```python
from build123d import *

# Parameters (mm, degrees)
SKETCH1_R           = 8
BOSS_EXTRUDE1_DEPTH = 55.781202295
BOSS_EXTRUDE2_DEPTH = 7.5
SKETCH4_W           = 9
SKETCH4_H           = 15
FILLET7_R           = 7.5


with BuildPart() as part:
    # Sketch1 → Boss-Extrude1 (new body)
    with BuildSketch(Plane.XY):
        with Locations(Location((0, 0, 0), (0, 0, 180))):
            Circle(SKETCH1_R)
    extrude(amount=BOSS_EXTRUDE1_DEPTH)

    # Sketch2 → Boss-Extrude2 (add, symmetric)
    with BuildSketch(Plane(origin=(0, 0, 0), x_dir=(1, 0, 0), z_dir=(0, 1, 0))):
        with BuildLine():
            Line((0, 0), (0, -47.781202295))
            Line((0, -47.781202295), (-8, -47.781202295))
            ThreePointArc((-8, -47.781202295), (-15.893349065, -27.087541453), (-35.563103488, -16.907496293))
            ThreePointArc((-35.563103488, -16.907496293), (-57.085036764, -8.603159393), (-71.811764706, 9.152941176))
            Line((-71.811764706, 9.152941176), (-78.588235294, 23.647058824))
            ThreePointArc((-78.588235294, 23.647058824), (-71.352941176, 43.588235294), (-51.411764706, 36.352941176))
            ThreePointArc((-51.411764706, 36.352941176), (-34.542879643, 17.146903418), (-10, 10))
            Line((-10, 10), (0, 10))
            Line((0, 10), (0, 0))
        make_face()
        with BuildLine():
            Line((-66.918339779, 28.396886626), (-50.887206037, 9.213488831))
            ThreePointArc((-50.887206037, 9.213488831), (-47.365752883, 8.898262426), (-47.050526478, 12.41971558))
            Line((-47.050526478, 12.41971558), (-63.081660221, 31.603113374))
            ThreePointArc((-63.081660221, 31.603113374), (-66.603113374, 31.918339779), (-66.918339779, 28.396886626))
        make_face(mode=Mode.SUBTRACT)
    extrude(amount=BOSS_EXTRUDE2_DEPTH, both=True)

    # Sketch4 → Cut-Revolve1 (revolve, cut)
    with BuildSketch(Plane(origin=(0, 0, 0), x_dir=(1, 0, 0), z_dir=(0, 1, 0))):
        with Locations((-4.5, -63.281202295)):
            Rectangle(SKETCH4_W, SKETCH4_H)
        with Locations((-4.5, 7.5)):
            Rectangle(SKETCH4_W, SKETCH4_H)
    revolve(axis=Axis((0, 0, 0), (0, 0, 1)), mode=Mode.SUBTRACT)

    # Fillet7
    # the kernel refuses this fillet: 7.5 mm, written as the material it takes off along each edge
    with BuildSketch(Plane(origin=(-10, -7.5, -10), x_dir=(0, 1, 0), z_dir=(1, 0, 0))) as fillet7_piece_1:
        with BuildLine():
            CenterArc((FILLET7_R, FILLET7_R), FILLET7_R, 180, 90)
            Line((0, FILLET7_R), (0, 0))
            Line((0, 0), (FILLET7_R, 0))
        make_face()
    extrude(amount=23.775062814, mode=Mode.SUBTRACT)
    with BuildSketch(Plane(origin=(-10, -7.5, -55.714285714), x_dir=(-0.9058823529411765, 0, 0.423529411764706), z_dir=(-0.423529411764706, 0, -0.9058823529411765))) as fillet7_piece_2:
        with BuildLine():
            CenterArc((45.714285714 + FILLET7_R, FILLET7_R), FILLET7_R, 180, 90)
            Line((45.714285714 + FILLET7_R, 0), (45.714285714, 0))
            Line((45.714285714, 0), (45.714285714, FILLET7_R))
        make_face()
    revolve(axis=Axis((-10, -7.5, -55.714285714), (0, 1, 0)), revolution_arc=64.942384582, mode=Mode.SUBTRACT)
    with BuildSketch(Plane(origin=(-65, -7.5, -30), x_dir=(-0.9058823529411761, 0, 0.42352941176470665), z_dir=(0.42352941176470665, 0, 0.9058823529411761))) as fillet7_piece_3:
        with BuildLine():
            CenterArc((15 - FILLET7_R, -FILLET7_R), FILLET7_R, 0, 90)
            Line((15 - FILLET7_R, 0), (15, 0))
            Line((15, 0), (15, -FILLET7_R))
        make_face()
    revolve(axis=Axis((-65, -7.5, -30), (0, -1, 0)), revolution_arc=180, mode=Mode.SUBTRACT)
    with BuildSketch(Plane(origin=(-71.811764706, -7.5, -9.152941176), x_dir=(0, 1, 0), z_dir=(-0.4235294117647053, 0, -0.9058823529411768))) as fillet7_piece_4:
        with BuildLine():
            CenterArc((FILLET7_R, FILLET7_R), FILLET7_R, 180, 90)
            Line((0, FILLET7_R), (0, 0))
            Line((0, 0), (FILLET7_R, 0))
        make_face()
    extrude(amount=16, mode=Mode.SUBTRACT)
    with BuildSketch(Plane(origin=(-30.4, -7.5, -28.514285714), x_dir=(-0.11294288879485842, 0, 0.9936014814152967), z_dir=(0.9936014814152967, 0, 0.11294288879485842))) as fillet7_piece_5:
        with BuildLine():
            CenterArc((45.714285714 - FILLET7_R, -FILLET7_R), FILLET7_R, 0, 90)
            Line((45.714285714 - FILLET7_R, 0), (45.714285714, 0))
            Line((45.714285714, 0), (45.714285714, -FILLET7_R))
        make_face()
    revolve(axis=Axis((-30.4, -7.5, -28.514285714), (0, -1, 0)), revolution_arc=58.45739638, mode=Mode.SUBTRACT)
    with BuildSketch(Plane(origin=(-10, 7.5, -10), x_dir=(0, -1, 0), z_dir=(1, 0, 0))) as fillet7_piece_6:
        with BuildLine():
            CenterArc((FILLET7_R, -FILLET7_R), FILLET7_R, 90, 90)
            Line((0, -FILLET7_R), (0, 0))
            Line((0, 0), (FILLET7_R, 0))
        make_face()
    extrude(amount=23.775062814, mode=Mode.SUBTRACT)
    with BuildSketch(Plane(origin=(-10, 7.5, -55.714285714), x_dir=(-0.9058823529411765, 0, 0.423529411764706), z_dir=(-0.423529411764706, 0, -0.9058823529411765))) as fillet7_piece_7:
        with BuildLine():
            CenterArc((45.714285714 + FILLET7_R, -FILLET7_R), FILLET7_R, 90, 90)
            Line((45.714285714 + FILLET7_R, 0), (45.714285714, 0))
            Line((45.714285714, 0), (45.714285714, -FILLET7_R))
        make_face()
    revolve(axis=Axis((-10, 7.5, -55.714285714), (0, 1, 0)), revolution_arc=64.942384582, mode=Mode.SUBTRACT)
    with BuildSketch(Plane(origin=(-65, 7.5, -30), x_dir=(-0.9058823529411761, 0, 0.42352941176470665), z_dir=(0.42352941176470665, 0, 0.9058823529411761))) as fillet7_piece_8:
        with BuildLine():
            CenterArc((15 - FILLET7_R, FILLET7_R), FILLET7_R, 270, 90)
            Line((15 - FILLET7_R, 0), (15, 0))
            Line((15, 0), (15, FILLET7_R))
        make_face()
    revolve(axis=Axis((-65, 7.5, -30), (0, -1, 0)), revolution_arc=180, mode=Mode.SUBTRACT)
    with BuildSketch(Plane(origin=(-71.811764706, 7.5, -9.152941176), x_dir=(0, -1, 0), z_dir=(-0.4235294117647053, 0, -0.9058823529411768))) as fillet7_piece_9:
        with BuildLine():
            CenterArc((FILLET7_R, -FILLET7_R), FILLET7_R, 90, 90)
            Line((0, -FILLET7_R), (0, 0))
            Line((0, 0), (FILLET7_R, 0))
        make_face()
    extrude(amount=16, mode=Mode.SUBTRACT)
    with BuildSketch(Plane(origin=(-30.4, 7.5, -28.514285714), x_dir=(-0.11294288879485842, 0, 0.9936014814152967), z_dir=(0.9936014814152967, 0, 0.11294288879485842))) as fillet7_piece_10:
        with BuildLine():
            CenterArc((45.714285714 - FILLET7_R, FILLET7_R), FILLET7_R, 270, 90)
            Line((45.714285714 - FILLET7_R, 0), (45.714285714, 0))
            Line((45.714285714, 0), (45.714285714, FILLET7_R))
        make_face()
    revolve(axis=Axis((-30.4, 7.5, -28.514285714), (0, -1, 0)), revolution_arc=58.45739638, mode=Mode.SUBTRACT)
    with BuildSketch(Plane(origin=(-39.072524125, -7.5, 47.781202295), x_dir=(0.8232772833721975, 0, 0.5676394231228962), z_dir=(-0.5676394231228962, 0, 0.8232772833721975))) as fillet7_piece_11_section:
        with BuildLine():
            CenterArc((31.072524125 + FILLET7_R, FILLET7_R), FILLET7_R, 180, 90)
            Line((31.072524125 + FILLET7_R, 0), (31.072524125, 0))
            Line((31.072524125, 0), (31.072524125, FILLET7_R))
        make_face()
    fillet7_piece_11 = revolve(axis=Axis((-39.072524125, -7.5, 47.781202295), (0, 1, 0)), revolution_arc=118.100790846, mode=Mode.PRIVATE)
    fillet7_piece_11 = fillet7_piece_11 - Plane(origin=(0, 0, 57.650012674), x_dir=(-1, 0, 0), z_dir=(0, 0, -1)) * Cylinder(8, 155, mode=Mode.PRIVATE)
    add(fillet7_piece_11, mode=Mode.SUBTRACT)
    with BuildSketch(Plane(origin=(-39.072524125, 7.5, 47.781202295), x_dir=(0.8232772833721975, 0, 0.5676394231228962), z_dir=(-0.5676394231228962, 0, 0.8232772833721975))) as fillet7_piece_12_section:
        with BuildLine():
            CenterArc((31.072524125 + FILLET7_R, -FILLET7_R), FILLET7_R, 90, 90)
            Line((31.072524125 + FILLET7_R, 0), (31.072524125, 0))
            Line((31.072524125, 0), (31.072524125, -FILLET7_R))
        make_face()
    fillet7_piece_12 = revolve(axis=Axis((-39.072524125, 7.5, 47.781202295), (0, 1, 0)), revolution_arc=118.100790846, mode=Mode.PRIVATE)
    fillet7_piece_12 = fillet7_piece_12 - Plane(origin=(0, 0, 57.650012673), x_dir=(-1, 0, 0), z_dir=(0, 0, -1)) * Cylinder(8, 155, mode=Mode.PRIVATE)
    add(fillet7_piece_12, mode=Mode.SUBTRACT)


solid = part.part
```
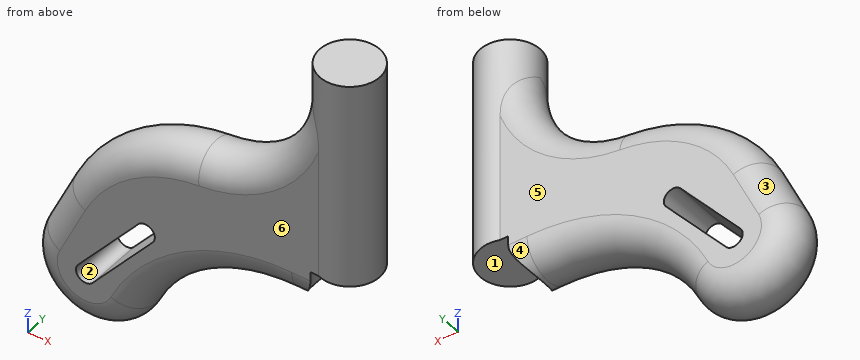
Could you check a few things on this model? Use its own coordinates, in mm. Face numbers are marked on the shaded views. A direction names the side the tool comes from. Coordinates: 2 decimals unless noted, no trailing zeros. Write each loop counter-clockwise with the first axis right and the second up, starting at its lowest first coordinate (ties: lowest second). Pieces come first, ordered by that corner, then holes. Notation, with made-up numbers: (-28.75, -24.5) -> (6.25, -24.5) arc R30 cw to (6.25, 4.5) -> close; hole circle Ø5 at (-34.75, -27.5). An arc over 180 degrees is marked (long way). Write item = value, one per line. Start each with the question number.
(1) Which directions (+Z, -Z, +X, -X, +Y, -Y) give clear straight access to the entire face, cutting with the end or side of a thin tool? Please do the marked faces 4, 5 and 6.
(2) I need wall thicknesses on line 1 (Y direction, x = -69, z = -25); line 2 (Z direction, x = -55, y = 3.25) (3 decimals); line 3 (Z direction, x = -62, y = -3.5). Which ranges of each line are inside material? Lowest first, please. Write a range as [from, to].
(3) I want a section at C-C (y = 6). Please give me the cut outline in (x, z).
(4) I want a section at A-A (y = 0). Please give me the cut outline in (x, z).
(5) I want a section at B-B (x = 0). Please give me the cut outline in (y, z), plus the area to 4 significant figures.
(6) Will these pins go through, and if not, where does the flat tip stop? pin 1 (4 mm diameter, centred on x = -56, y = -2.5, fed in from -Z); pin 2 (6 mm diameter, centred on y = -3.5, z = 1, fed in from -X); pin 3 (3 mm diameter, centred on x = -16, y = -4.5, fed in from -Z).
(7) We'd pull the mould along Z, two halves only. Please class the marked faces 1, 2 and 3: released by +Z, released by -Z, zero draft, split by the parting line, or undercut.
Result set:
q1.face_4 = -Z, +X
q1.face_5 = +Z, -Z, -X, +Y
q1.face_6 = +Z, -Z, -X, -Y
q2.line_1 = [-7.5, 7.5]
q2.line_2 = [-40.165, -21.932], [-14.135, 9.135]
q2.line_3 = [-43.81, -30.31], [-22.51, 3.31]
q3.outline = (-75.87, -24.92) arc R12 ccw to (-54.13, -35.08) arc R48.71 cw to (-10, -7) -> (-6.71, -7) -> (-6.71, 0) -> (5.29, 0) -> (5.29, 55.78) -> (-5.29, 55.78) -> (-5.29, 43.33) arc R34.07 cw to (-35.22, 13.93) arc R42.71 ccw to (-69.09, -10.42) -> close; hole (-66.92, -28.4) arc R2.5 ccw to (-63.08, -31.6) -> (-47.05, -12.42) arc R2.5 ccw to (-50.89, -9.21) -> close
q4.outline = (-78.59, -23.65) arc R15 ccw to (-51.41, -36.35) arc R45.71 cw to (-10, -10) -> (-9, -10) -> (-9, 0) -> (8, 0) -> (8, 55.78) -> (-8, 55.78) -> (-8, 47.78) arc R31.07 cw to (-35.56, 16.91) arc R45.71 ccw to (-71.81, -9.15) -> close; hole (-66.92, -28.4) arc R2.5 ccw to (-63.08, -31.6) -> (-47.05, -12.42) arc R2.5 ccw to (-50.89, -9.21) -> close
q5.outline = (-8, 0) -> (8, 0) -> (8, 55.78) -> (-8, 55.78) -> close
q5.area = 892.5 mm2
q6.pin_1 = -42.95
q6.pin_2 = -67.02
q6.pin_3 = -9.79
q7.face_1 = released by -Z
q7.face_2 = undercut
q7.face_3 = released by +Z
